```python
from build123d import *

# Parameters (mm, degrees)
SKETCH1_R           = 12.7
BOSS_EXTRUDE1_DEPTH = 254
SKETCH2_W           = 50.8
SKETCH2_H           = 31.75
BOSS_EXTRUDE2_DEPTH = 63.5
CUT_EXTRUDE1_REACH  = 52.8
SKETCH3_W           = 57.15
SKETCH3_H           = 25.4


with BuildPart() as part:
    # Sketch1 → Boss-Extrude1 (new body)
    with BuildSketch(Plane.XY):
        Circle(SKETCH1_R)
    extrude(amount=BOSS_EXTRUDE1_DEPTH)

    # Sketch2 → Boss-Extrude2 (add)
    with BuildSketch(Plane.XY.offset(254)):
        Rectangle(SKETCH2_W, SKETCH2_H)
    extrude(amount=BOSS_EXTRUDE2_DEPTH)

    # Sketch3 → Cut-Extrude1 (cut, up to next)
    with BuildSketch(Plane(origin=(25.4, 0, 0), x_dir=(0, 0, -1), z_dir=(1, 0, 0)), mode=Mode.PRIVATE) as cut_extrude1_sk1:
        with Locations((-288.925, 3.175)):
            Rectangle(SKETCH3_W, SKETCH3_H)
    cut_extrude1_tool1 = extrude(cut_extrude1_sk1.sketch, amount=-CUT_EXTRUDE1_REACH, mode=Mode.PRIVATE) & part.part
    add(cut_extrude1_tool1.solids().sort_by_distance((25.4, 3.175, 288.925))[0], mode=Mode.SUBTRACT)


solid = part.part
```
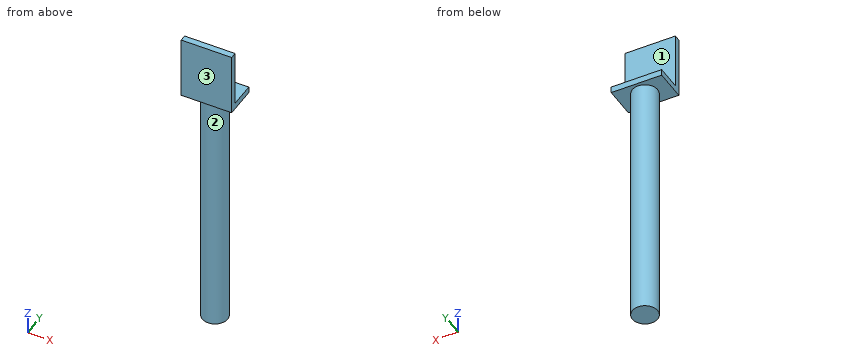
Model file for the job. Use its own axes, mm. Face numbers are marked on the shaded views. A direction names the side the tool comes from. Give positions to 0.01 mm unless a question says otherwise; leave off trailing zeros. Write each loop counter-clockwise with the first axis right and the second up, starting at its lowest first coordinate (ties: lowest second). Pieces come first, ordered by that corner, then holes. Notation, with made-up numbers: (-3, -24.5) - (14, -24.5) arc R9 ccw to (14, -8.5) - close; hole circle Ø7 at (-27, 62.5). An arc over 180 degrees is marked (long way). One line per question, with ' | ' between items. Start each with the question number.
(1) 3-axis set-ups, long thin cutter, end or side, ignore diameter. For the marked faces 1, 2 and 3: which of +Z, -Z, +X, -X, +Y, -Y reach the whole face in a straight line?
(2) Slice it at C-C on z = 297. Write the cut outline in (x, y) (3 decimals).
(3) Wall check: line 1 along Z through (x, y) = (-16, 11); line 2 along X through (y, z) = (0.5, 124); line 3 along Z through (x, y) = (17, -12.5). Give the ranges that are in metal, low to high. Write a range as from..to.
(4) Slice it at A-A on y = 0. Write the cut outline in (x, z).
(5) Slice it at B-B on x = 16. Write the cut outline in (y, z) (3 decimals).
(6) Pin check, flat tips, straight feed: P1, Ø1, axis at x = -0.5, z = 76.5, coming from the -Y side; P2, Ø8, axis at y = -3, z = 153.5, coming from the -X side; P3, Ø6, axis at x = 14.5, z = 193.5, coming from the -Y side. Stop position of each tip, or through.
(7) Slice it at D-D on x = 0. Write the cut outline in (y, z) (3 decimals).
Results below:
1) face 1: +Z, +X, -X, +Y | face 2: -Z | face 3: +Z, -Z, +X, -X, -Y
2) outline: (-25.4, -15.875) - (25.4, -15.875) - (25.4, -9.525) - (-25.4, -9.525) - close
3) line 1: 254..260.35 | line 2: -12.69..12.69 | line 3: 254..317.5
4) outline: (-25.4, 254) - (-12.7, 254) - (-12.7, 0) - (12.7, 0) - (12.7, 254) - (25.4, 254) - (25.4, 260.35) - (-25.4, 260.35) - close
5) outline: (-15.875, 254) - (15.875, 254) - (15.875, 260.35) - (-9.525, 260.35) - (-9.525, 317.5) - (-15.875, 317.5) - close
6) P1: y = -12.7 | P2: x = -12.7 | P3: y = -5.39
7) outline: (-15.875, 254) - (-12.7, 254) - (-12.7, 0) - (12.7, 0) - (12.7, 254) - (15.875, 254) - (15.875, 260.35) - (-9.525, 260.35) - (-9.525, 317.5) - (-15.875, 317.5) - close
